from build123d import *

# Parameters (mm, degrees)
SKETCH_1_W          = 45
SKETCH_1_H          = 35
EXTRUDE_1_DEPTH     = 5
SKETCH_2_W          = 6
SKETCH_2_H          = 35
EXTRUDE_2_DEPTH     = 45
SKETCH_3_R          = 3
CUT_EXTRUDE_1_DEPTH = 70.507193872
FILLET_1_R          = 3
FILLET_2_R          = 4
CUT_EXTRUDE_2_REACH = 59.554
SKETCH_4_R          = 2


with BuildPart() as part:
    # 草图1 → 凸台-拉伸1 (new body)
    with BuildSketch(Plane.XY):
        Rectangle(SKETCH_1_W, SKETCH_1_H)
    extrude(amount=EXTRUDE_1_DEPTH)

    # 草图2 → 凸台-拉伸2 (add)
    with BuildSketch(Plane.XY.offset(5)):
        with Locations((-19.5, 0)):
            Rectangle(SKETCH_2_W, SKETCH_2_H)
    extrude(amount=EXTRUDE_2_DEPTH)

    # 草图3 → 切除-拉伸1 (cut, through all)
    with BuildSketch(Plane.ZY.offset(22.5)):
        with Locations((30, 0)):
            Circle(SKETCH_3_R)
    extrude(amount=-CUT_EXTRUDE_1_DEPTH, mode=Mode.SUBTRACT)

    # 圆角1
    fillet_1_edges = [part.edges().sort_by_distance(p)[0] for p in [
        (22.5, -17.5, 2.5),
        (22.5, 17.5, 2.5),
    ]]
    fillet(fillet_1_edges, radius=FILLET_1_R)

    # 圆角2
    fillet_2_edges = [part.edges().sort_by_distance(p)[0] for p in [
        (-19.5, -17.5, 50),
        (-19.5, 17.5, 50),
    ]]
    fillet(fillet_2_edges, radius=FILLET_2_R)

    # 草图4 → 切除-拉伸2 (cut, up to next)
    with BuildSketch(Plane(origin=(0, 0, 0), x_dir=(-1, 0, 0), z_dir=(0, 0, -1)), mode=Mode.PRIVATE) as cut_extrude_2_sk1:
        with Locations((-13, 10)):
            Circle(SKETCH_4_R)
    cut_extrude_2_tool1 = extrude(cut_extrude_2_sk1.sketch, amount=-CUT_EXTRUDE_2_REACH, mode=Mode.PRIVATE) & part.part
    # 草图4 → 切除-拉伸2 (cut, up to next)
    with BuildSketch(Plane(origin=(0, 0, 0), x_dir=(-1, 0, 0), z_dir=(0, 0, -1)), mode=Mode.PRIVATE) as cut_extrude_2_sk2:
        with Locations((13, 10)):
            Circle(SKETCH_4_R)
    cut_extrude_2_tool2 = extrude(cut_extrude_2_sk2.sketch, amount=-CUT_EXTRUDE_2_REACH, mode=Mode.PRIVATE) & part.part
    # 草图4 → 切除-拉伸2 (cut, up to next)
    with BuildSketch(Plane(origin=(0, 0, 0), x_dir=(-1, 0, 0), z_dir=(0, 0, -1)), mode=Mode.PRIVATE) as cut_extrude_2_sk3:
        with Locations((13, -10)):
            Circle(SKETCH_4_R)
    cut_extrude_2_tool3 = extrude(cut_extrude_2_sk3.sketch, amount=-CUT_EXTRUDE_2_REACH, mode=Mode.PRIVATE) & part.part
    # 草图4 → 切除-拉伸2 (cut, up to next)
    with BuildSketch(Plane(origin=(0, 0, 0), x_dir=(-1, 0, 0), z_dir=(0, 0, -1)), mode=Mode.PRIVATE) as cut_extrude_2_sk4:
        with Locations((-13, -10)):
            Circle(SKETCH_4_R)
    cut_extrude_2_tool4 = extrude(cut_extrude_2_sk4.sketch, amount=-CUT_EXTRUDE_2_REACH, mode=Mode.PRIVATE) & part.part
    add(cut_extrude_2_tool1.solids().sort_by_distance((13, 10, 0))[0], mode=Mode.SUBTRACT)
    add(cut_extrude_2_tool2.solids().sort_by_distance((-13, 10, 0))[0], mode=Mode.SUBTRACT)
    add(cut_extrude_2_tool3.solids().sort_by_distance((-13, -10, 0))[0], mode=Mode.SUBTRACT)
    add(cut_extrude_2_tool4.solids().sort_by_distance((13, -10, 0))[0], mode=Mode.SUBTRACT)


solid = part.part
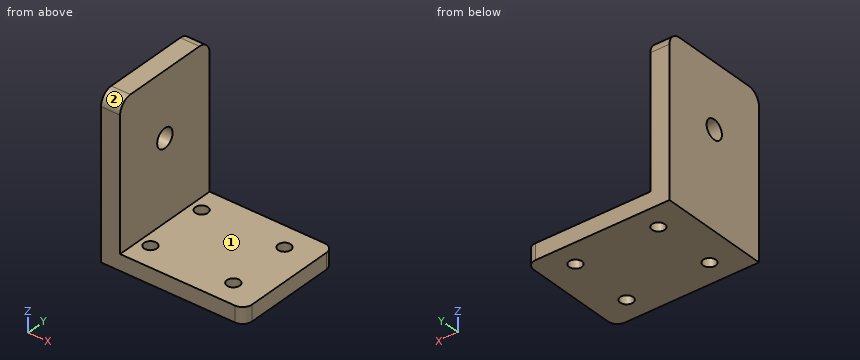
Can you work these out from the model? Positions are in its coordinate system, mm. Face numbers are marked on the shaded views. A direction names the side the tool comes from. Coordinates: 2 decimals unless noted, no trailing zeros. Write each loop counter-clockwise with the first axis right and the second up, starting at its lowest first coordinate (ties: lowest second). Pieces come first, ordered by that corner, then holes. Notation, with made-up numbers: (-2, 34.5) - (33, 34.5) arc R25 ccw to (33, 53.5) - close; hole circle Ø11 at (-10.5, 8). An arc over 180 degrees is marked (long way). Return JSON: item names as keys, results as strings. Group by question number.
Item 1: If we section it at D-D (z = 30): Write out the boundary of the cut face in (x, y).
Item 2: Which directions (+Z, -Z, +X, -X, +Y, -Y) give clear straight access to the entire face, cutting with the end or side of a thin tool? Please do the marked faces 1 and 2.
Item 3: Please list where these lines run through material, in increasing order: probe 1 along Y at (x, z) = (-13, 3.45); probe 2 along Y at (x, z) = (-20.55, 30); probe 3 along Z at (x, y) = (19.5, -14).
Item 4: If we section it at A-A (x = -13): Write out the boundary of the cut face in (y, z).
Item 5: If we section it at C-C (y = 10): Write out the boundary of the cut face in (x, z), then the cut area to 3 significant figures.
Item 6: If we section it at B-B (y = 0): Write out the boundary of the cut face in (x, z).
Item 7: I'm going to push flat-ended pins straight in: pin 1 Ø12 at (x, z) = (7, 6.5) entering from -Y; pin 2 Ø4.5 at (x, y) = (13, 10) entering from +Z; pin 3 Ø8 at (y, z) = (-8.5, 32) entering from +X. Where does each tip first touch, or does it pass through?
Return value:
{
 "1": {"outline": "(-22.5, -17.5) - (-16.5, -17.5) - (-16.5, -3) - (-22.5, -3) - close; (-22.5, 3) - (-16.5, 3) - (-16.5, 17.5) - (-22.5, 17.5) - close"},
 "2": {"face 1": "+Z, +X, +Y, -Y", "face 2": "+Z, +X, -X, -Y"},
 "3": {"probe 1": "y = -17.5 to -12, -8 to 8, 12 to 17.5", "probe 2": "y = -17.5 to -3, 3 to 17.5", "probe 3": "z = 0 to 5"},
 "4": {"outline": "(-17.5, 0) - (-12, 0) - (-12, 5) - (-17.5, 5) - close; (-8, 0) - (8, 0) - (8, 5) - (-8, 5) - close; (12, 0) - (17.5, 0) - (17.5, 5) - (12, 5) - close"},
 "5": {"outline": "(-22.5, 0) - (-15, 0) - (-15, 5) - (-16.5, 5) - (-16.5, 50) - (-22.5, 50) - close; (-11, 0) - (11, 0) - (11, 5) - (-11, 5) - close; (15, 0) - (22.5, 0) - (22.5, 5) - (15, 5) - close", "area": "455 mm^2"},
 "6": {"outline": "(-22.5, 0) - (22.5, 0) - (22.5, 5) - (-16.5, 5) - (-16.5, 27) - (-22.5, 27) - close; (-22.5, 33) - (-16.5, 33) - (-16.5, 50) - (-22.5, 50) - close"},
 "7": {"pin 1": "stops at y = -17.5", "pin 2": "stops at z = 5", "pin 3": "stops at x = -16.5"}
}
